Can you work these out from the model? Positions are in its coordinate system, mm. A direction names the side the tool comes from. Coordinates: 2 decimals unless noted, no trailing zeros. Order: outer loops, then holes, each group sorted by start corner. A loop starts at its lowest first (then second) coordinate and runs counter-clockwise, first axis right, second up. Notation, with made-up numbers: (7.5, 72) -> (23.5, 72) arc R13 cw to (23.5, 87) -> close; hole circle Ø9 at (39.5, 34.5). An arc over 180 degrees is marked (long way). Use a Markdown table: item, result. Add a question column.
1. If I drill on line 1 along X through (y, z) = (0, -0.25); line 2 along Y through (x, z) = (7.25, -9.5); line 3 along X through (y, z) = (-3.25, -12.5), over which ranges is the centre line in solid material (lowest first)? Write a range as from..to.
2. Suppose I cut it at A-A, the plane y = 0. List the corners of the cut face in (x, z) for me.
3. Suppose I cut it at B-B, the plane z = -3. List the corners of the cut face in (x, y) for me.
4. For faces 5 (the flat face through (0, 0, 0)), 6 (the flat face through (-2.5, 2.5, -0.5)), 7 (the flat face through (2.3, 2.3, -12.8)), which set-ups out of +Z, -Z, +X, -X, +Y, -Y let a thin tool reach every point of the face, with its end or its side?
5. We'd pull the mould along Y, two halves only. Please class faces 1 (the conical face through (7.078, 3.965, -9.303)), 2 (the cylindrical face through (-3, 0, -13)), 3 (the conical face through (0.106, 8.112, -9.303)), 4 (the flat face through (-1, -1, -13.3)): pulls with the +Y half, pulls with the -Y half, needs draft (parallel to the pull), parting line crosses it, or undercut.
6. For pin 1 Ø2.5 at (x, y) = (-7.14, -4.12) entering from -Z; pin 2 Ø1.5 at (x, y) = (-6, -6) entering from +Z; pin 3 Ø1 at (x, z) = (0.5, -16) entering from -Y; pin 4 Ø4 at (x, z) = (-9.5, -15) entering from -Y, each with a flat end and sliding along its axis, tell me the tip position at first contact or that it passes through.
```python
from build123d import *

# Parameters (mm, degrees)
SKETCH2_R           = 1
BOSS_EXTRUDE1_DEPTH = 6
CIRPATTERN1_COUNT   = 6


with BuildPart() as part:
    # Sketch1 → Revolve1 (revolve)
    with BuildSketch(Plane(origin=(0, 0, 0), x_dir=(1, 0, 0), z_dir=(0, 1, 0))):
        with BuildLine():
            Line((0, 0), (3, 0))
            Line((3, 0), (3, 0.5))
            Line((3, 0.5), (11.9, 0.5))
            Line((11.9, 0.5), (11.9, 0))
            Line((11.9, 0), (12.2, 0))
            Line((12.2, 0), (12.2, 11.8))
            ThreePointArc((12.2, 11.8), (11.907106781, 12.507106781), (11.2, 12.8))
            Line((11.2, 12.8), (3, 12.8))
            Line((3, 12.8), (3, 13.3))
            Line((3, 13.3), (0, 13.3))
            Line((0, 13.3), (0, 0))
        make_face()
    revolve(axis=Axis((0, 0, 0), (0, 0, -1)))

    # Sketch2 → Boss-Extrude1 (add)
    with BuildSketch(Plane(origin=(0, 0, -13.3), x_dir=(-1, 0, 0), z_dir=(0, 0, -1))):
        Circle(SKETCH2_R)
    extrude(amount=BOSS_EXTRUDE1_DEPTH)

    # Sketch4 → M1.6 Clearance Hole1 (revolve, cut)
    with BuildSketch(Plane(origin=(0, 8.25, -12.8), x_dir=(0, 1, 0), z_dir=(1, 0, 0))):
        Polygon((0, 0), (0, 3.600860619), (1, 3), (1, 0), align=None)
    m1_6_clearance_hole1 = revolve(axis=Axis((0, 8.25, -19.15), (0, 0, 1)), mode=Mode.SUBTRACT)

    # CirPattern1: M1.6 Clearance Hole1 ×6 about axis
    cirpattern1_axis = Axis((0, 0, 0), (0, 0, 1))
    for i in range(1, CIRPATTERN1_COUNT):
        add(m1_6_clearance_hole1.rotate(cirpattern1_axis, i * 360 / CIRPATTERN1_COUNT), mode=Mode.SUBTRACT)


solid = part.part
```
Worked out:
| question | item | result |
|---|---|---|
| 1 | line 1 | x = -12.2..-11.9, -3..3, 11.9..12.2 |
| 1 | line 2 | y = -9.81..-4.61, -3.64..3.64, 4.61..9.81 |
| 1 | line 3 | x = -11.46..-7.63, -6.66..6.66, 7.63..11.46 |
| 2 | outline | (-12.2, -11.8) arc R1 ccw to (-11.2, -12.8) -> (-3, -12.8) -> (-3, -13.3) -> (-1, -13.3) -> (-1, -19.3) -> (1, -19.3) -> (1, -13.3) -> (3, -13.3) -> (3, -12.8) -> (11.2, -12.8) arc R1 ccw to (12.2, -11.8) -> (12.2, 0) -> (11.9, 0) -> (11.9, -0.5) -> (3, -0.5) -> (3, 0) -> (-3, 0) -> (-3, -0.5) -> (-11.9, -0.5) -> (-11.9, 0) -> (-12.2, 0) -> close |
| 3 | outline | circle Ø24.4 at (0, 0) |
| 4 | face 5 | +Z, +X, -X, +Y, -Y |
| 4 | face 6 | +Z |
| 4 | face 7 | -Z |
| 5 | face 1 | undercut |
| 5 | face 2 | parting line crosses it |
| 5 | face 3 | undercut |
| 5 | face 4 | needs draft |
| 6 | pin 1 | stops at z = -12.8 |
| 6 | pin 2 | stops at z = -0.5 |
| 6 | pin 3 | stops at y = -1 |
| 6 | pin 4 | passes through |
